from build123d import *

# Parameters (mm, degrees)
F0_W     = 176.5
F0_H     = 195
F1_DEPTH = 68.3
F2_R     = 5
F3_DEPTH = 3
F4_R     = 6
F5_DEPTH = 25


with BuildPart() as f1:
    # F0 (on Top) → F1 (new body)
    with BuildSketch(Plane.XY):
        with Locations((-88.25, 97.5)):
            Rectangle(F0_W, F0_H)
    extrude(amount=-F1_DEPTH)

    # F2 (on face) → F3 (join)
    with BuildSketch(Plane.XY):
        with Locations((-25, 170)):
            Circle(F2_R)
        with Locations((-151.5, 170)):
            Circle(F2_R)
        with Locations((-151.5, 25)):
            Circle(F2_R)
        with Locations((-25, 25)):
            Circle(F2_R)
    extrude(amount=F3_DEPTH)

    # F4 (on face) → F5 (cut)
    with BuildSketch(Plane.YZ):
        with Locations((143.3, -49)):
            Circle(F4_R)
        with Locations((113.3, -49)):
            Circle(F4_R)
        with Locations((83.3, -49)):
            Circle(F4_R)
        with Locations((53.3, -49)):
            Circle(F4_R)
        with Locations((53.3, -20)):
            Circle(F4_R)
        with Locations((83.3, -20)):
            Circle(F4_R)
        with Locations((113.3, -20)):
            Circle(F4_R)
        with Locations((143.3, -20)):
            Circle(F4_R)
    extrude(amount=-F5_DEPTH, mode=Mode.SUBTRACT)


solid = f1.part
Read the model definition and answer for the solid it produces. Units are mm, in the model's axes. A direction names the side the tool comes from. Give positions to 0.01 mm unless a question says otherwise; leave off trailing zeros. Loops run counter-clockwise (first coordinate to the right, second up) from the corner with the lowest first, then second, coordinate; pieces in that order, holes last. Notation, with made-up numbers: M 86,36 L 133,36 A30 ccw 133,64 Z; hole C 30,73.25 d8. An arc over 180 degrees is marked long. Write each question's results on one line, items separated by ' | '.
1. Straight lines are drawn through the part: line 1 (Z direction, x = -16.25, y = 83.3); line 2 (Y direction, x = -22, z = -24); line 3 (X direction, y = 147, z = -48). For each, find the intervals that lie inside material, in ascending order. Write a range as [from, to].
Values:
line 1: z = [-68.3, -55], [-43, -26], [-14, 0] | line 2: y = [0, 48.83], [57.77, 78.83], [87.77, 108.83], [117.77, 138.83], [147.77, 195] | line 3: x = [-176.5, -25]
2. Given pin 1 (11 mm diameter, centred on y = 83.3, z = -49, fed in from +X); pin 2 (1.5 mm diameter, centred on x = -129.5, y = 30.5, fed in from +Z), each flat-ended and moving along its own axis, determine where each tip first touches the part or whether it passes through.
Values:
pin 1: stops at x = -25 | pin 2: stops at z = 0
3. A tool of negligible diameter and unlimited length cuts with its end or side. For faces 1 (the face through (-12.325, 77.306, -48.736)), 2 (the face through (-152.151, 174.957, 1.479)), 3 (the face through (-89, 99, -68.3)), from which of +Z, -Z, +X, -X, +Y, -Y can it reach the whole face along a straight path? Write none if from no direction.
Values:
face 1: +X | face 2: +Z | face 3: -Z, +X, -X, +Y, -Y
4. Section A-A on x = -151.5 is taken. Give the vertices of the cut face in (y, z), plus the area to 3 significant figures.
Values:
outline: M 0,-68.3 L 195,-68.3 L 195,0 L 175,0 L 175,3 L 165,3 L 165,0 L 30,0 L 30,3 L 20,3 L 20,0 L 0,0 Z | area: 13,400 mm^2
5. The mould has two halves that part along X. Classify faces 4 (the face through (-25, 53, -49)), 5 (the face through (-25.651, 174.957, 1.479)), 6 (the face through (-12.32, 58.84, -51.3)): pulls with the +X half, pulls with the -X half, needs draft (parallel to the pull), parting line crosses it, or undercut.
Values:
face 4: pulls with the +X half | face 5: undercut | face 6: needs draft
6. Section B-B on y = 25 is taken. Give the vertices of the cut face in (x, z).
Values:
outline: M -176.5,-68.3 L 0,-68.3 L 0,0 L -20,0 L -20,3 L -30,3 L -30,0 L -146.5,0 L -146.5,3 L -156.5,3 L -156.5,0 L -176.5,0 Z
7. Section D-D on x = -83 is taken. Give the vertices of the cut face in (y, z), plus the area to 3 significant figures.
Values:
outline: M 0,-68.3 L 195,-68.3 L 195,0 L 0,0 Z | area: 13,300 mm^2
8. Section C-C on z = -20 is taken. Give the vertices of the cut face in (x, y), plus the area to 3 significant figures.
Values:
outline: M -176.5,0 L 0,0 L 0,47.3 L -25,47.3 L -25,59.3 L 0,59.3 L 0,77.3 L -25,77.3 L -25,89.3 L 0,89.3 L 0,107.3 L -25,107.3 L -25,119.3 L 0,119.3 L 0,137.3 L -25,137.3 L -25,149.3 L 0,149.3 L 0,195 L -176.5,195 Z | area: 33,200 mm^2
